```python
from build123d import *

# Parameters (mm, degrees)
SKETCH2_R               = 2.05
CUT_EXTRUDE1_DEPTH      = 40.350070343
BOSS_EXTRUDE2_DEPTH     = 4.394
CUT_EXTRUDE2_DEPTH      = 40.350070343
CUT_EXTRUDE2_DEPTH_BACK = 40.350070343


with BuildPart() as part:
    # Sketch1 → Revolve1 (revolve)
    with BuildSketch(Plane(origin=(0, 0, 0), x_dir=(1, 0, 0), z_dir=(0, 1, 0)), mode=Mode.PRIVATE) as revolve1_sk:
        Polygon((-15.875, 0), (-27.5, 0), (-27.5, -5.994), (-16.075, -5.994), (-16.075, -4.394), (-15.875, -4.394), align=None)
    revolve(revolve1_sk.sketch.rotate(Axis((0, 0, 1.024477222), (0, 0, -1)), 180), axis=Axis((0, 0, 1.024477222), (0, 0, -1)))

    # Sketch2 → Cut-Extrude1 (cut, through all)
    with BuildSketch(Plane.XY):
        with Locations((-15.556349186, 15.556349186)):
            Circle(SKETCH2_R)
        with Locations((15.556349186, 15.556349186)):
            Circle(SKETCH2_R)
        with Locations((15.556349186, -15.556349186)):
            Circle(SKETCH2_R)
        with Locations((-15.556349186, -15.556349186)):
            Circle(SKETCH2_R)
    extrude(amount=CUT_EXTRUDE1_DEPTH, mode=Mode.SUBTRACT)

    # Sketch3 → Boss-Extrude2 (add)
    with BuildSketch(Plane(origin=(0, 0, 0), x_dir=(-1, 0, 0), z_dir=(0, 0, -1))):
        with BuildLine():
            ThreePointArc((-10.642530671, 11.779310927), (-15.76562668, -1.860279655), (-7.608598211, -13.932869707))
            Line((-7.608598211, -13.932869707), (-7.189226656, -13.164916258))
            ThreePointArc((-7.189226656, -13.164916258), (-14.89665513, -1.757744556), (-10.055934492, 11.130057569))
            Line((-10.055934492, 11.130057569), (-10.642530671, 11.779310927))
        make_face()
        with BuildLine():
            Line((7.924235053, -13.755803278), (7.487466192, -12.997609396))
            ThreePointArc((7.487466192, -12.997609396), (4.450525747, -14.324553067), (1.196324742, -14.952217465))
            Line((1.196324742, -14.952217465), (1.266110352, -15.82443015))
            ThreePointArc((1.266110352, -15.82443015), (4.710139749, -15.160151996), (7.924235053, -13.755803278))
        make_face()
        with BuildLine():
            Line((9.110684324, -11.916183582), (9.642140909, -12.611294291))
            ThreePointArc((9.642140909, -12.611294291), (12.705557645, -9.517585299), (14.81331567, -5.708003492))
            Line((14.81331567, -5.708003492), (13.996833704, -5.393389127))
            ThreePointArc((13.996833704, -5.393389127), (12.005251319, -8.992993983), (9.110684324, -11.916183582))
        make_face()
        with BuildLine():
            ThreePointArc((9.362835646, 12.820020814), (5.987616034, 14.702519486), (2.257535542, 15.713661517))
            Line((2.257535542, 15.713661517), (2.133104449, 14.847554189))
            ThreePointArc((2.133104449, 14.847554189), (5.657589953, 13.892144396), (8.846773838, 12.113405494))
            Line((8.846773838, 12.113405494), (9.362835646, 12.820020814))
        make_face()
    extrude(amount=-BOSS_EXTRUDE2_DEPTH)

    # Sketch4 → Cut-Extrude2 (cut, two sides: drawn at the far end of the back side and taken through both)
    with BuildSketch(Plane(origin=(0, 0, 0), x_dir=(-1, 0, 0), z_dir=(0, 0, -1)).offset(-CUT_EXTRUDE2_DEPTH_BACK)):
        with BuildLine():
            Line((-8.963010633, -13.680627024), (0, 0))
            Line((0, 0), (-2.655754961, -16.138218023))
            ThreePointArc((-2.655754961, -16.138218023), (-5.937917721, -15.239299476), (-8.963010633, -13.680627024))
        make_face()
    extrude(amount=CUT_EXTRUDE2_DEPTH + CUT_EXTRUDE2_DEPTH_BACK, mode=Mode.SUBTRACT)


solid = part.part
```
For this review, take the finished solid that the model builds, in its own axes (mm). A direction names the side the tool comes from. Coordinates: 2 decimals unless noted, no trailing zeros. Loops run counter-clockwise (first coordinate to the right, second up) from the corner with the lowest first, then second, coordinate; pieces in that order, holes last.
1. Add section D-D, the plane y = 22. Give the boundary of the cut face in (x, z), then the cut area to 3 significant figures.
2. For faces 1 (the flat face through (12, -9.5, 4.394)), 2 (the flat face through (-12, -12, 0)), 3 (the cylindrical face through (-15.27, 4.34, 2.17)), list the 3-axis set-ups (+Z, -Z, +X, -X, +Y, -Y) from which the entire face can be reached by the end or side of a thin tool; tool diameter is ignored.
3. For line 1 (X direction, y = -0.5, z = 5.5); line 2 (Y direction, x = 0, z = 5) (3 decimals); line 3 (Y direction, x = -6, z = 4.3), list the stretches that pass through material, from the lowest coordinate up.
4. Add section B-B, the plane x = 0. Give the boundary of the cut face in (y, z) (3 decimals), then the cut area to 3 significant figures.
5. Mouldability with a two-part tool opening along X and no side actions: class faces 4 (the flat face through (12, 12, 5.994)), 5 (the cylindrical face through (12.69, 24.397, 3.039)), 6 (the cylindrical face through (15.112, 13.555, 2.955)) as +X half, -X half, draft (parallel to the pull), parting line (faces both ways), or undercut.
6. Insertion check: P1, Ø10, axis at x = 9, y = -12.5, coming from the +Z side; P2, Ø2, axis at y = -2.5, z = 4, coming from the +X side; P3, Ø2, axis at y = -12.5, z = 5, coming from the -X side; P4, Ø1, axis at y = 9.5, z = 4, coming from the -X side. Each pin has a flat end and moves straight along its axis. Give the tip position at first contact, or say it passes through.
7. Add section C-C, the plane z = 1.4. Give the boundary of the cut face in (x, y) (3 decimals), then the cut area to 3 significant figures.
8. Add section A-A, the plane y = 0. Give the boundary of the cut face in (x, z) (3 decimals).
Result:
1. outline: (-16.5, 0) - (16.5, 0) - (16.5, 5.99) - (-16.5, 5.99) - close
1. area: 198 mm2
2. face 1: +Z
2. face 2: -Z, +X, -X, +Y, -Y
2. face 3: +Z, -Z
3. line 1: x = -27.5 to -16.07, 16.07 to 27.5
3. line 2: y = -27.5 to -16.075, 16.075 to 27.5
3. line 3: y = -26.84 to -13.75, 13.75 to 26.84
4. outline: (-27.5, 0) - (-15.875, 0) - (-15.875, 4.394) - (-16.075, 4.394) - (-16.075, 5.994) - (-27.5, 5.994) - close; (15.875, 0) - (27.5, 0) - (27.5, 5.994) - (16.075, 5.994) - (16.075, 4.394) - (15.875, 4.394) - close
4. area: 139 mm2
5. face 4: draft
5. face 5: parting line
5. face 6: undercut
6. P1: stops at z = 5.99
6. P2: stops at x = 27.46
6. P3: stops at x = -24.98
6. P4: stops at x = -25.99
7. outline: circle Ø55 at (0, 0); hole circle Ø4.1 at (-15.556, -15.556); hole circle Ø4.1 at (-15.556, 15.556); hole (-14.813, -5.708) - (-13.997, -5.393) arc R15 ccw to (-9.111, -11.916) - (-9.642, -12.611) arc R15.875 ccw to (-7.924, -13.756) - (-7.487, -12.998) arc R15 ccw to (-1.196, -14.952) - (-1.266, -15.824) arc R15.875 ccw to (2.578, -15.664) - (2.656, -16.138) arc R16.355 ccw to (8.963, -13.681) - (8.22, -12.547) arc R15 ccw to (10.056, 11.13) - (10.643, 11.779) arc R15.875 ccw to (-2.258, 15.714) - (-2.133, 14.848) arc R15 ccw to (-8.847, 12.113) - (-9.363, 12.82) arc R15.875 ccw to start; hole circle Ø4.1 at (15.556, -15.556); hole circle Ø4.1 at (15.556, 15.556)
7. area: 1,570 mm2
8. outline: (-27.5, 0) - (-15.875, 0) - (-15.875, 4.394) - (-16.075, 4.394) - (-16.075, 5.994) - (-27.5, 5.994) - close; (15, 0) - (27.5, 0) - (27.5, 5.994) - (16.075, 5.994) - (16.075, 4.394) - (15, 4.394) - close
